Source: CAD feature listing. Evaluate the final solid. Frame: model axes, mm. Face numbers are marked on the shaded views. A direction names the side the tool comes from. Coordinates: 2 decimals unless noted, no trailing zeros. Order: outer loops, then holes, each group sorted by start corner. A loop starts at its lowest first (then second) coordinate and runs counter-clockwise, first axis right, second up.
```python
from build123d import *

# Parameters (mm, degrees)
SKETCH_R  = 1.6
PAD_DEPTH = 4
FILLET_R  = 2


with BuildPart() as part:
    # Sketch → Pad (new body)
    with BuildSketch(Plane.XY):
        Polygon((0, 22.5), (12, 22.5), (12, -22.5), (0, -22.5), (0, -25), (-13, -25), (-13, 25), (0, 25), align=None)
        with Locations((6, 10)):
            Circle(SKETCH_R, mode=Mode.SUBTRACT)
        with Locations((6, -10)):
            Circle(SKETCH_R, mode=Mode.SUBTRACT)
        with Locations((-6.5, 20)):
            Circle(SKETCH_R, mode=Mode.SUBTRACT)
        with Locations((-6.5, 12)):
            Circle(SKETCH_R, mode=Mode.SUBTRACT)
    extrude(amount=PAD_DEPTH)

    # Fillet
    fillet_edges = [part.edges().sort_by_distance(p)[0] for p in [
        (12, 22.5, 2),
        (0, 25, 2),
        (-13, 25, 2),
        (-13, -25, 2),
        (0, -25, 2),
        (12, -22.5, 2),
    ]]
    fillet(fillet_edges, radius=FILLET_R)


solid = part.part
```
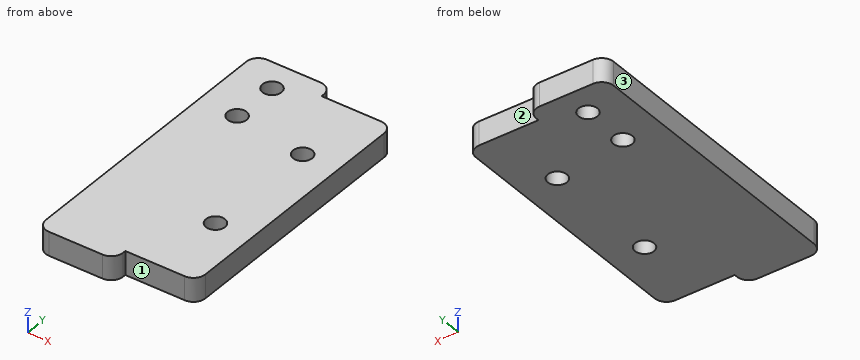
Q1. Set-up query: the marked faces 1, 2 and 3. Return all of +Z, -Z, +X, -X, +Y, -Y with unobstructed straight access to the full face (end or side cutting, diameter ignored); none if empty.
Solutions:
face 1: +Z, -Z, +X, -Y
face 2: +Z, -Z, +X, +Y
face 3: +Z, -Z, -X, +Y, -Y
Q2. Section query C-C on y = 21. Output: boundary loops of the cut face in (x, z).
Solutions:
outline: (-13, 0) - (-7.75, 0) - (-7.75, 4) - (-13, 4) - close; (-5.25, 0) - (11.94, 0) - (11.94, 4) - (-5.25, 4) - close
Q3. Section query A-A on x = 6. Output: boundary loops of the cut face in (y, z), plus the area to 3 significant figures.
Solutions:
outline: (-22.5, 0) - (-11.6, 0) - (-11.6, 4) - (-22.5, 4) - close; (-8.4, 0) - (8.4, 0) - (8.4, 4) - (-8.4, 4) - close; (11.6, 0) - (22.5, 0) - (22.5, 4) - (11.6, 4) - close
area: 154 mm2
Q4. Pin query (flat end, axial travel): P1, Ø2, axis at x = 7, z = 2, coming from the -Y side; P2, Ø0.6, axis at y = 22.5, z = 2.5, coming from the +X side; P3, Ø5, axis at x = 6, y = -10, coming from the +Z side; P4, Ø1, axis at x = 3, z = 1.5, coming from the +Y side. Return the tip coordinate at first contact, or that it passes through.
Solutions:
P1: stops at y = -22.5
P2: stops at x = 11.05
P3: stops at z = 4
P4: stops at y = 22.5
Q5. Section query D-D on x = -6.5. Output: boundary loops of the cut face in (y, z), plus the area to 3 significant figures.
Solutions:
outline: (-25, 0) - (10.4, 0) - (10.4, 4) - (-25, 4) - close; (13.6, 0) - (18.4, 0) - (18.4, 4) - (13.6, 4) - close; (21.6, 0) - (25, 0) - (25, 4) - (21.6, 4) - close
area: 174 mm2
Q6. Material intervals for line 1 along Y through (x, z) = (-6.5, 3.05); line 2 along Y through (x, z) = (5, 1.9); line 3 along Y through (x, z) = (2.25, 3), sorted ascending.
Solutions:
line 1: y = -25 to 10.4, 13.6 to 18.4, 21.6 to 25
line 2: y = -22.5 to -11.25, -8.75 to 8.75, 11.25 to 22.5
line 3: y = -22.5 to 22.5
Q7. Section query B-B on z = 1.55. Output: boundary loops of the cut face in (x, y), plus the area to 3 significant figures.
Solutions:
outline: (-13, -23) arc R2 ccw to (-11, -25) - (-2, -25) arc R2 ccw to (0, -23) - (0, -22.5) - (10, -22.5) arc R2 ccw to (12, -20.5) - (12, 20.5) arc R2 ccw to (10, 22.5) - (0, 22.5) - (0, 23) arc R2 ccw to (-2, 25) - (-11, 25) arc R2 ccw to (-13, 23) - close; hole circle Ø3.2 at (-6.5, 12); hole circle Ø3.2 at (-6.5, 20); hole circle Ø3.2 at (6, -10); hole circle Ø3.2 at (6, 10)
area: 1,150 mm2
